Geometry check sheet. Reference: the model listing, model coordinates, mm. A direction names the side the tool comes from. Coordinates: 2 decimals unless noted, no trailing zeros. Order: outer loops, then holes, each group sorted by start corner. A loop starts at its lowest first (then second) coordinate and runs counter-clockwise, first axis right, second up. Notation, with made-up numbers: (17.25, 27.25) - (62.25, 27.25) arc R23 ccw to (62.25, 60.25) - close; hole circle Ø7 at (48, -29.75). An arc over 180 degrees is marked (long way). Put each result on its own line as item: value.
from build123d import *

# Parameters (mm, degrees)
SKETCH_1_R          = 40
SKETCH_1_R_2        = 35.15
EXTRUDE_1_DEPTH     = 28.5
SKETCH_2_R          = 35.5
SKETCH_2_R_2        = 29
EXTRUDE_2_DEPTH     = 5
SKETCH_3_R          = 50
SKETCH_3_R_2        = 40
EXTRUDE_3_DEPTH     = 5
SKETCH_4_R          = 1.6
CUT_EXTRUDE_1_DEPTH = 75.51342161
FILLET_1_R          = 1.5
FILLET_2_R          = 2


with BuildPart() as part:
    # 草图1 → 凸台-拉伸1 (new body)
    with BuildSketch(Plane.XY):
        with Locations(Location((0, 0, 0), (0, 0, 180))):
            Circle(SKETCH_1_R)
        with Locations(Location((0, 0, 0), (0, 0, 180))):
            Circle(SKETCH_1_R_2, mode=Mode.SUBTRACT)
    extrude(amount=EXTRUDE_1_DEPTH)

    # 草图2 → 凸台-拉伸2 (add)
    with BuildSketch(Plane.XY.offset(28.5)):
        Circle(SKETCH_2_R)
        Circle(SKETCH_2_R_2, mode=Mode.SUBTRACT)
    extrude(amount=-EXTRUDE_2_DEPTH)

    # 草图3 → 凸台-拉伸3 (add)
    with BuildSketch(Plane(origin=(0, 0, 0), x_dir=(-1, 0, 0), z_dir=(0, 0, -1))):
        Circle(SKETCH_3_R)
        Circle(SKETCH_3_R_2, mode=Mode.SUBTRACT)
    extrude(amount=-EXTRUDE_3_DEPTH)

    # 草图4 → 切除-拉伸1 (cut, through all)
    with BuildSketch(Plane.XY.offset(5)):
        with Locations((31.819805153, 31.819805153)):
            Circle(SKETCH_4_R)
        with Locations((31.819805153, -31.819805153)):
            Circle(SKETCH_4_R)
        with Locations((-31.819805153, -31.819805153)):
            Circle(SKETCH_4_R)
        with Locations((-31.819805153, 31.819805153)):
            Circle(SKETCH_4_R)
        with Locations((0, 45)):
            Circle(SKETCH_4_R)
        with Locations((0, -45)):
            Circle(SKETCH_4_R)
    extrude(amount=-CUT_EXTRUDE_1_DEPTH, mode=Mode.SUBTRACT)

    # 圆角1
    fillet_1_edges = [part.edges().sort_by_distance(p)[0] for p in [
        (35.15, 0, 23.5),
        (40, 0, 28.5),
    ]]
    fillet(fillet_1_edges, radius=FILLET_1_R)

    # 圆角2
    fillet_2_edges = [part.edges().sort_by_distance(p)[0] for p in [
        (-29, 0, 23.5),
    ]]
    fillet(fillet_2_edges, radius=FILLET_2_R)


solid = part.part
Q1. Section check B-B on x = 0. State how many separate pieces and enclosed holes the cut face has, then the cut area to 3 significant figures.
Answer block:
separate pieces: 4
enclosed holes: 0
area: 404 mm^2
Q2. Draft check along Y on faces 3 (the cylindrical face through (0.74, 43.58, 2.54)), 4 (the cylindrical face through (39.96, -1.76, 15.85)), 5 (the flat face through (10, -30, 23.5)), 6 (the flat face through (15, 37.3, 5)). Enter one of: pulls with the +Y half, pulls with the -Y half, needs draft (parallel to the pull), parting line crosses it, or undercut.
Answer block:
face 3: undercut
face 4: parting line crosses it
face 5: undercut
face 6: needs draft
Q3. Thickness scan on L1, parallel to Y at x = 0, z = 2.15; L2, parallel to Y at x = 0, z = 26.6; L3, parallel to Z at x = -15.5, y = 40.5. Record the ranges inside material, lowest first. Write a range as [from, to].
Answer block:
L1: y = [-50, -46.6], [-43.4, -35.15], [35.15, 43.4], [46.6, 50]
L2: y = [-40, -29], [29, 40]
L3: z = [0, 5]
Q4. Depth check by flat-ended pin: pin 1 Ø12 at (x, z) = (10.5, 13) entering from +Y; pin 2 Ø5 at (y, z) = (18, 21) entering from +X; pin 3 Ø12 at (x, z) = (-4.5, 18) entering from +Y; pin 4 Ø10 at (x, y) = (35.5, -32) entering from -Z. Enter the tip coordinate at first touch or a pass-through.
Answer block:
pin 1: stops at y = 39.75
pin 2: stops at x = 36.87
pin 3: stops at y = 40
pin 4: stops at z = 0
Q5. Access from +Z, -Z, +X, -X, +Y, -Y to the whole of each face (thin tool, end or side, straight path). Record for faces 1 (the cylindrical face through (-47.69, 15.02, 2.46)), 2 (the cylindrical face through (-33.527, -10.558, 10.846)).
Answer block:
face 1: +Z, -Z
face 2: -Z
Q6. Section check D-D on y = 45. Record the boundary of the cut face in (x, z).
Answer block:
outline: (-21.79, 0) - (-1.6, 0) - (-1.6, 5) - (-21.79, 5) - close; (1.6, 0) - (21.79, 0) - (21.79, 5) - (1.6, 5) - close
Q7. Section check A-A on y = 0. Record the boundary of the cut face in (x, z).
Answer block:
outline: (-50, 0) - (-35.15, 0) - (-35.15, 22) arc R1.5 cw to (-33.65, 23.5) - (-31, 23.5) arc R2 ccw to (-29, 25.5) - (-29, 28.5) - (-38.5, 28.5) arc R1.5 ccw to (-40, 27) - (-40, 5) - (-50, 5) - close; (29, 25.5) arc R2 ccw to (31, 23.5) - (33.65, 23.5) arc R1.5 cw to (35.15, 22) - (35.15, 0) - (50, 0) - (50, 5) - (40, 5) - (40, 27) arc R1.5 ccw to (38.5, 28.5) - (29, 28.5) - close
Q8. Section check C-C on z = 3. Record the boundary of the cut face in (x, y), then the cut area to 3 significant figures.
Answer block:
outline: circle Ø100 at (0, 0); hole circle Ø70.3 at (0, 0); hole circle Ø3.2 at (-31.82, -31.82); hole circle Ø3.2 at (-31.82, 31.82); hole circle Ø3.2 at (0, -45); hole circle Ø3.2 at (0, 45); hole circle Ø3.2 at (31.82, -31.82); hole circle Ø3.2 at (31.82, 31.82)
area: 3,920 mm^2
